Model file for the job. Use its own axes, mm. A direction names the side the tool comes from. Give positions to 0.01 mm unless a question says otherwise; leave off trailing zeros. Order: outer loops, then holes, each group sorted by start corner. A loop starts at its lowest first (then second) coordinate and runs counter-clockwise, first axis right, second up. Notation, with made-up numbers: M 4,44 L 20,44 A19 cw 20,63 Z; hole C 85,69.25 d1. An arc over 180 degrees is marked long. Return JSON: item names as keys, results as strings. Group by question number.
1. Slice it at B-B on y = 79. List the corners of the cut face in (x, z), then the cut area to 3 significant figures.
2. 3-axis set-ups, long thin cutter, end or side, ignore diameter. For faces 1 (the face through (52.081, 30.685, 2.535)), 2 (the face through (77.81, 70, 2)), 3 (the face through (116.81, 70, 3)): which of +Z, -Z, +X, -X, +Y, -Y reach the whole face in a straight line?
3. Slice it at C-C on x = 88. List the corners of the cut face in (y, z), then the cut area to 3 significant figures.
4. Pin check, flat tips, straight feed: pin 1 (3 mm diameter, centred on y = 73, z = 2.5, fed in from -X); pin 2 (1 mm diameter, centred on x = 89, z = 3.5, fed in from -Y); pin 3 (2.5 mm diameter, centred on x = 51.5, z = 1.5, fed in from +Y). Stop position of each tip, or through.
5. Wall check: probe 1 along X at (y, z) = (50.5, 3.8); probe 2 along Y at (x, z) = (92.5, 3.45); probe 3 along X at (y, z) = (35, 1.1). Give the ranges that are in metal, low to high. Write a range as [from, to].
6. Two-plate mould, pull along Y, no slides. Class faces 4 (the face through (81.759, 35.565, 2.535)), 5 (the face through (58, 50, 2)), 6 (the face through (84.34, 30.39, 2.54)), 7 (the face through (77.81, 95, 3)): released by +Y, released by -Y, zero draft, split by the parting line, or undercut.
7. Slice it at A-A on z = 1.3. List the corners of the cut face in (x, y).
Autodesk Inventor part; units mm, degrees
ref_plane "YZ Plane" through (0, 0, 0) normal (1, 0, 0) x (0, 1, 0)
ref_plane "XZ Plane" through (0, 0, 0) normal (0, 1, 0) x (-1, 0, 0)
ref_plane "XY Plane" through (0, 0, 0) normal (0, 0, 1) x (1, 0, 0)
sketch "Sketch2" plane through (0, 0, 0) normal (0, 0, 1) x (1, 0, 0)
  line L0 (0, 0) -> (100, 0)
  line L1 (100, 0) -> (100, 100)
  line L2 (100, 100) -> (0, 100)
  line L3 (0, 100) -> (0, 0)
  dimension "d24" = 100
  dimension "d25" = 100
extrude "Extrusion3" add sketch "Sketch2" along normal blind 5
sketch "Sketch3" plane through (0, 0, 5) normal (0, 0, 1) x (1, 0, 0)
  line L0 (100, 100) -> (0, 100)
  line L1 (61.1065, 16.5645) -> (65.8098, 9.5096)
  ellipse E0 centre (57.8098, 14.5814) end of major axis (53.8097, 14.5816) minor radius 3.4641
  line L2 (49.8098, 9.5096) -> (54.5131, 16.5645)
  line L3 (65.8098, 9.5096) -> (77.2764, 15.2429)
  line L4 (83.9156, 31.2525) -> (78.0026, 43.0784)
  line L5 (49.8098, 26.1436) -> (54.4159, 35.3558)
  line L6 (58.3112, 37.4887) -> (58.6416, 37.4249)
  line L7 (56.9769, 37.4324) -> (57.4131, 37.502)
  line L8 (38.6658, 33.573) -> (49.8098, 26.1436)
  ellipse E1 centre (30.5481, 100.1015) end of major axis (25.0287, 91.7624) minor radius 10.0002
  line L9 (78.4473, 33.7186) -> (83.2584, 30.5112)
  line L10 (83.2584, 30.5112) -> (84.5136, 29.6744)
  line L11 (83.9156, 31.2525) -> (84.7776, 29.4984)
  line L12 (83.9156, 31.2525) -> (85.87, 31.2525) construction
  line L13 (84.7776, 29.4984) -> (84.5136, 29.6744)
  line L14 (78.4473, 33.7186) -> (77.8098, 34.1436)
  line L15 (78.4473, 33.7186) -> (79.931, 33.7186) construction
  line L16 (77.2128, 33.7456) -> (77.8098, 34.1436)
  line L17 (77.2128, 33.7456) -> (77.9303, 33.7456) construction
  line L18 (57.8098, 14.5814) -> (57.8098, 100)
  arc A0 (47.8099, 100) -> (37.8097, 90) centre (47.8099, 89.9998) ccw
  line L19 (47.8099, 89.9998) -> (57.8098, 89.9998)
  line L20 (57.8098, 89.9998) -> (67.8098, 89.9998)
  line L21 (57.8098, 89.9998) -> (67.8098, 89.9998) construction
  arc A1 (77.81, 90) -> (67.8098, 100) centre (67.8098, 89.9998) ccw
  line L22 (47.8099, 100) -> (67.8098, 100)
  line L23 (78.0026, 43.0784) -> (77.81, 43.4636)
  line L24 (78.0026, 43.0784) -> (78.4334, 43.0784) construction
  line L25 (77.81, 43.4636) -> (77.81, 43.8508)
  line L26 (65.8098, 26.1436) -> (61.2037, 35.3558)
  line L27 (37.8097, 63.9104) -> (37.8098, 35.2913)
  line L28 (38.6658, 33.573) -> (37.8098, 34.1436)
  line L29 (38.6658, 33.573) -> (39.6945, 33.573) construction
  line L30 (37.8098, 34.1436) -> (37.8098, 35.2913)
  line L31 (37.8097, 63.9104) -> (37.8097, 90)
  arc A2 (61.2037, 35.3558) -> (54.4159, 35.3558) centre (57.8098, 35.2913) ccw
  line L32 (65.8098, 26.1436) -> (77.2128, 33.7456)
  line L33 (77.81, 43.8508) -> (77.81, 90)
  line L34 (100, 0) -> (100, 100)
  line L35 (0, 100) -> (100, 100)
  line L36 (100, 100) -> (100, 0)
  line L37 (100, 0) -> (0, 0)
  line L38 (0, 0) -> (0, 100)
  point P0 (78.3106, 15.3544)
  point P1 (77.7245, 15.3467)
  point P2 (77.3127, 15.2462)
  point P3 (60.1591, 36.6399)
  point P4 (55.4604, 36.6398)
  point P5 (91.0098, 173.4299)
  dimension "d31" = 296.17
  dimension "d32" = 213.69
  dimension "d33" = 326.31
  dimension "d34" = 10
  dimension "d35" = 0
  dimension "d36" = 243.43
  dimension "d37" = 213.69
extrude "Extrusion4" cut sketch "Sketch3" against normal blind 10 contours E0 | L34 L37 L38 L0 E1 A0 L31 L27 L30 L28 L8 L5 A2 L26 L32 L16 L14 L9 L10 L13 L11 L4 L23 L25 L33 A1 | A0 E1 L0 | E1 L0 picked at (31.1987, 94.7741)
ref_plane "Work Plane2" through (49.8098, 26.1436, 5) normal (0, -0.433, -0.9014) x (-1, 0, 0)
ref_plane "Work Plane1" through (100, 100, 0) normal (0, -0.433, -0.9014) x (-1, 0, 0)
sketch "Sketch4" plane through (49.8098, 26.1436, 5) normal (0, -0.433, -0.9014) x (-1, 0, 0)
  line L0 (-27.403, 9.0174) -> (-16, 2.1651)
  line L1 (-16, 2.1651) -> (-27.403, 9.0174)
  point P0 (49.8098, -21.4002)
sketch "Sketch5" plane through (77.81, 43.4636, 5) normal (1, 0, 0) x (0, 0, -1)
  line L0 (5, 46.5364) -> (5, 56.5364)
  line L1 (5, 56.5364) -> (0, 56.5364)
  line L2 (0, 56.5364) -> (0, -3.4636)
  line L3 (0, -3.4636) -> (5, -3.4636)
  line L4 (5, -3.4636) -> (5, 56.5364)
  point P0 (5, -43.4636)
  dimension "d41" = 5
  dimension "d42" = 60
extrude "Extrusion5" add sketch "Sketch5" along normal blind 39
sketch "Sketch6" plane through (0, 0, 0) normal (0, 0, -1) x (-1, 0, 0)
  line L0 (-37.8097, 100) -> (-77.8097, 100)
  line L1 (-77.8097, 100) -> (-77.8097, 50)
  line L2 (-77.8097, 50) -> (-37.8097, 50)
  line L3 (-37.8097, 50) -> (-37.8097, 100)
  point P0 (0, 0)
  dimension "d45" = 40
  dimension "d46" = 50
extrude "Extrusion6" cut sketch "Sketch6" against normal blind 5
properties part number "Arm_Base"
Result:
{
 "1": {"outline": "M 77.81,0 L 116.81,0 L 116.81,5 L 77.81,5 Z", "area": "195 mm2"},
 "2": {"face 1": "+Z, -Z, -Y", "face 2": "+Z, -Z, -X, +Y", "face 3": "+Z, -Z, +X, +Y, -Y"},
 "3": {"outline": "M 40,0 L 100,0 L 100,5 L 40,5 Z", "area": "300 mm2"},
 "4": {"pin 1": "stops at x = 77.81", "pin 2": "stops at y = 40", "pin 3": "stops at y = 50"},
 "5": {"probe 1": "x = [77.81, 116.81]", "probe 2": "y = [40, 100]", "probe 3": "x = [37.81, 54.24], [61.38, 82.04]"},
 "6": {"face 4": "undercut", "face 5": "released by +Y", "face 6": "undercut", "face 7": "zero draft"},
 "7": {"outline": "M 37.81,34.14 L 38.67,33.57 L 49.81,26.14 L 54.42,35.36 A3.39 cw 61.2,35.36 L 65.81,26.14 L 77.81,34.14 L 84.78,29.5 L 83.92,31.25 L 79.54,40 L 116.81,40 L 116.81,100 L 77.81,100 L 77.81,90 A10 ccw 77.81,90.08 L 77.81,50 L 37.81,50 L 37.81,35.29 Z"}
}
